Autodesk Inventor part; units mm, degrees
ref_plane "YZ Plane" through (0, 0, 0) normal (1, 0, 0) x (0, 1, 0)
ref_plane "XZ Plane" through (0, 0, 0) normal (0, 1, 0) x (-1, 0, 0)
ref_plane "XY Plane" through (0, 0, 0) normal (0, 0, 1) x (1, 0, 0)
sketch "Sketch1" plane through (0, 0, 0) normal (0, 0, 1) x (1, 0, 0)
  circle A0 centre (0, 0) radius 7.95
  dimension "d0" = 15.9
extrude "Extrusion1" add sketch "Sketch1" along normal blind 4.82
sketch "Sketch2" plane through (0, 0, 4.82) normal (0, 0, 1) x (1, 0, 0)
  circle A0 centre (0, 0) radius 7.95
  circle A1 centre (0, 0) radius 6
  dimension "d3" = 12
extrude "Extrusion2" add sketch "Sketch2" along normal blind 4.6 contours A1
sketch "Sketch3" plane through (0, 0, 9.42) normal (0, 0, 1) x (1, 0, 0)
  circle A0 centre (0, 0) radius 6
  circle A1 centre (0, 0) radius 7.95
  circle A2 centre (0, 0) radius 7.95
extrude "Extrusion3" add sketch "Sketch3" along normal blind 2.15 contours A0 | A1
sketch "Sketch4" plane through (0, 0, 11.57) normal (0, 0, 1) x (1, 0, 0)
  circle A0 centre (0, 0) radius 7.95
  circle A1 centre (0, 0) radius 6
  dimension "d8" = 12
extrude "Extrusion4" add sketch "Sketch4" along normal blind 15 contours A1
sketch "Sketch5" plane through (0, 0, 0) normal (0, 0, -1) x (-1, 0, 0)
  circle A0 centre (0, 0) radius 7.95
hole "Hole1" at (0, 0, 0) direction (0, 0, 1) diameter 4.917 end through all
properties part number "peek-insulator"
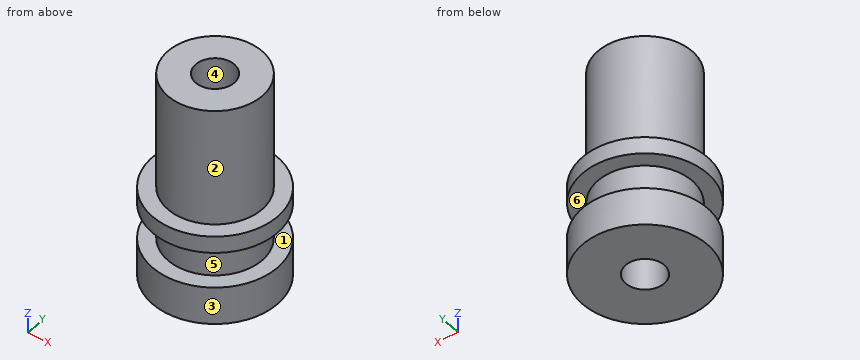
Could you check a few things on this model? Use its own coordinates, in mm. Face numbers are marked on the shaded views. A direction names the side the tool comes from. Coordinates: 2 decimals unless noted, no trailing zeros. Loops run counter-clockwise (first coordinate to the right, second up) from the corner with the lowest first, then second, coordinate; pieces in that order, holes last. Notation, with made-up numbers: M 26,78 L 62,78 A22 ccw 62,102 Z; hole C 71.5,53.5 d11. An arc over 180 degrees is marked long. Put each result on its own line as item: value. Start each with the question number.
(1) Suppose I cut it at A-A on x = 0. Please give me the cut outline in (y, z).
(2) Suppose I cut it at C-C on z = 14.5. Please give me the cut outline in (x, y).
(3) Thinking about a two-plate mould opening in Y: for the marked faces 4, 5 and 6, which applies, pulls with the +Y half, pulls with the -Y half, needs draft (parallel to the pull), parting line crosses it, or undercut?
(4) Suppose I cut it at D-D on x = -3.25. Please give me the cut outline in (y, z).
(5) Will these pins go through, and if not, where does the flat tip stop? P1, Ø5, axis at y = -4, z = 10.5, coming from the +X side; P2, Ø1, axis at y = 1.5, z = 16, coming from the +X side; P3, Ø2, axis at x = -6, y = -4, coming from the +Z side.
(6) For the marked faces 1, 2 and 3, which set-ups out of +Z, -Z, +X, -X, +Y, -Y let a thin tool reach every point of the face, with its end or its side?
(7) I need wall thicknesses on line 1 (Z direction, x = 6, y = -4.75); line 2 (Y direction, x = 0, z = 16); line 3 (Y direction, x = 0, z = 9.75). Which ranges of each line are inside material? Lowest first, please. Write a range as from..to.
Solutions:
1. outline: M -7.95,0 L -2.46,0 L -2.46,26.57 L -6,26.57 L -6,11.57 L -7.95,11.57 L -7.95,9.42 L -6,9.42 L -6,4.82 L -7.95,4.82 Z; M 2.46,0 L 7.95,0 L 7.95,4.82 L 6,4.82 L 6,9.42 L 7.95,9.42 L 7.95,11.57 L 6,11.57 L 6,26.57 L 2.46,26.57 Z
2. outline: C 0,0 d12; hole C 0,0 d4.92
3. face 4: undercut
3. face 5: parting line crosses it
3. face 6: needs draft
4. outline: M -7.26,0 L 7.26,0 L 7.26,4.82 L 5.04,4.82 L 5.04,9.42 L 7.26,9.42 L 7.26,11.57 L 5.04,11.57 L 5.04,26.57 L -5.04,26.57 L -5.04,11.57 L -7.26,11.57 L -7.26,9.42 L -5.04,9.42 L -5.04,4.82 L -7.26,4.82 Z
5. P1: stops at x = 7.81
5. P2: stops at x = 5.92
5. P3: stops at z = 11.57
6. face 1: none
6. face 2: +Z
6. face 3: +Z, -Z
7. line 1: z = 0..4.82, 9.42..11.57
7. line 2: y = -6..-2.46, 2.46..6
7. line 3: y = -7.95..-2.46, 2.46..7.95
